Could you check a few things on this drawing? It's one solid part, dimensions in mm from its lowest x, y, z. Give positions to 0.01 mm unless a question says otherwise; leave off trailing zeros. Order: outer loops, then holes, each group sorted by start corner. A loop starts at its lowest first (then second) coordinate and runs counter-clockwise, first axis right, second up. Notation, with made-up numbers: (30.5, -18) - (77.5, -18) arc R15 ccw to (77.5, -14) - close; hole circle Ø9 at (-4, 15). An arc over 180 degrees is marked (long way). Return JSON: item names as keys, results as strings.
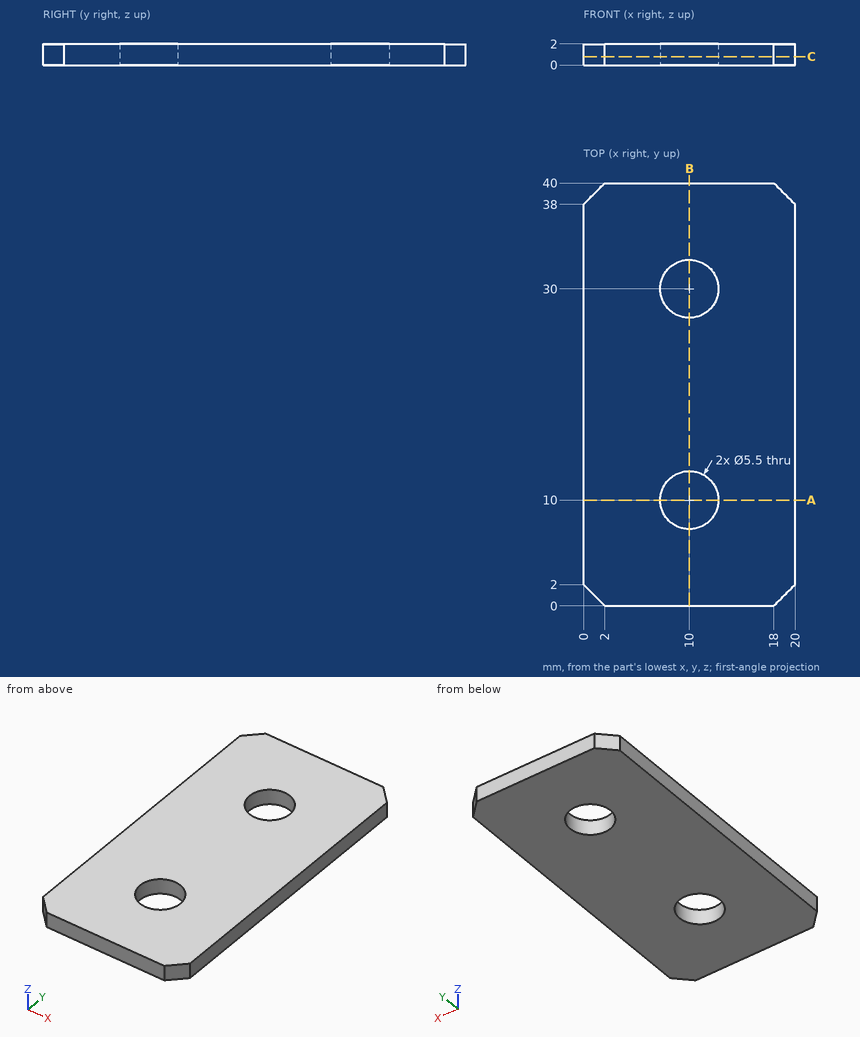
1. Suppose I cut it at C-C (z = 0.8). List the corners of the cut face in (x, y) for me, plus the area to 3 significant figures.
Checks:
{"outline": "(0, 2) - (2, 0) - (18, 0) - (20, 2) - (20, 38) - (18, 40) - (2, 40) - (0, 38) - close; hole circle Ø5.5 at (10, 10); hole circle Ø5.5 at (10, 30)", "area": "744 mm^2"}
2. If I drill on L1, parallel to Y at x = 10, z = 0.8; L2, parallel to Y at x = 12.25, z = 1; L3, parallel to X at y = 8, z = 0.1, over which ranges is the centre line in solid material (lowest first)? Write a range as [from, to].
Checks:
{"L1": "[0, 7.25], [12.75, 27.25], [32.75, 40]", "L2": "[0, 8.42], [11.58, 28.42], [31.58, 40]", "L3": "[0, 8.11], [11.89, 20]"}
3. Suppose I cut it at B-B (x = 10). List the corners of the cut face in (y, z) for me, plus the area to 3 significant figures.
Checks:
{"outline": "(0, 0) - (7.25, 0) - (7.25, 2) - (0, 2) - close; (12.75, 0) - (27.25, 0) - (27.25, 2) - (12.75, 2) - close; (32.75, 0) - (40, 0) - (40, 2) - (32.75, 2) - close", "area": "58.0 mm^2"}
4. Suppose I cut it at A-A (y = 10). List the corners of the cut face in (x, z) for me.
Checks:
{"outline": "(0, 0) - (7.25, 0) - (7.25, 2) - (0, 2) - close; (12.75, 0) - (20, 0) - (20, 2) - (12.75, 2) - close"}
5. For pin 1 Ø10 at (x, y) = (17.5, 21.5) entering from -Z, with a flat end and sliding along its axis, tell me the tip position at first contact or that it passes through.
Checks:
{"pin 1": "z = 0"}
